```python
from build123d import *

# Parameters (mm, degrees)
SKETCH1_R               = 12.5
SKETCH1_R_2             = 10
BOSS_EXTRUDE1_DEPTH     = 5
SKETCH2_W               = 28
SKETCH2_H               = 28
BOSS_EXTRUDE2_DEPTH     = 25
CUT_EXTRUDE1_DEPTH      = 29
SKETCH7_W               = 9.14199999
SKETCH7_H               = 19.416637146
CUT_EXTRUDE2_DEPTH      = 1
CUT_EXTRUDE2_DEPTH_BACK = 29
SKETCH8_R               = 3.5
CUT_EXTRUDE3_DEPTH      = 1
CUT_EXTRUDE3_DEPTH_BACK = 29


with BuildPart() as part:
    # Sketch1 → Boss-Extrude1 (new body)
    with BuildSketch(Plane.XY):
        Circle(SKETCH1_R)
        Circle(SKETCH1_R_2, mode=Mode.SUBTRACT)
    extrude(amount=BOSS_EXTRUDE1_DEPTH)

    # Sketch2 → Boss-Extrude2 (add)
    with BuildSketch(Plane.XY.offset(5)):
        Rectangle(SKETCH2_W, SKETCH2_H)
    extrude(amount=BOSS_EXTRUDE2_DEPTH)

    # Sketch3 → Cut-Extrude1 (cut, through all)
    with BuildSketch(Plane.ZY.offset(14)):
        with BuildLine():
            Line((17.5, 14), (30, 14))
            Line((30, 14), (30, -14))
            Line((30, -14), (17.5, -14))
            ThreePointArc((17.5, -14), (29.804652609, 0), (17.5, 14))
        make_face()
    extrude(amount=-CUT_EXTRUDE1_DEPTH, mode=Mode.SUBTRACT)

    # Sketch7 → Cut-Extrude2 (cut, two sides)
    with BuildSketch(Plane.XZ.offset(14)) as cut_extrude2_sk:
        with Locations((0, 21.203451283)):
            Rectangle(SKETCH7_W, SKETCH7_H)
    extrude(amount=CUT_EXTRUDE2_DEPTH, mode=Mode.SUBTRACT)
    extrude(cut_extrude2_sk.sketch, amount=-CUT_EXTRUDE2_DEPTH_BACK, mode=Mode.SUBTRACT)

    # Sketch8 → Cut-Extrude3 (cut, two sides)
    with BuildSketch(Plane(origin=(14, 0, 0), x_dir=(0, 0, -1), z_dir=(1, 0, 0))) as cut_extrude3_sk:
        with Locations((-23.652326304, 0)):
            Circle(SKETCH8_R)
    extrude(amount=CUT_EXTRUDE3_DEPTH, mode=Mode.SUBTRACT)
    extrude(cut_extrude3_sk.sketch, amount=-CUT_EXTRUDE3_DEPTH_BACK, mode=Mode.SUBTRACT)


solid = part.part
```
Design review of the part built by this model. Coordinates are the model's own, in mm. A direction names the side the tool comes from. Give positions to 0.01 mm unless a question says otherwise; leave off trailing zeros. Write each loop counter-clockwise with the first axis right and the second up, starting at its lowest first coordinate (ties: lowest second). Pieces come first, ordered by that corner, then holes. Notation, with made-up numbers: (5.5, 52) - (54.5, 52) arc R12 cw to (54.5, 64) - close; hole circle Ø10 at (78.25, 59). An arc over 180 degrees is marked (long way). Return JSON: item names as keys, results as strings. Group by question number.
(1) To check wall thickness, follow probe 1 along X at (y, z) = (7.5, 26.5); probe 2 along Y at (x, z) = (0, 2.4); probe 3 along Z at (x, y) = (4.5, 4.75). State the ranges of each line that lie inside material, in increasing order.
(2) We need section D-D, the plane x = 0. Give the boundary of the cut face in (y, z), then the cut area to 3 significant figures.
(3) We need section C-C, the plane z = 13.25. Give the boundary of the cut face in (x, y).
(4) Insertion check: pin 1 (1 mm diameter, centred on x = -1, y = 5, fed in from -Z); pin 2 (9 mm diameter, centred on y = -1, z = 25, fed in from -X); pin 3 (2.5 mm diameter, centred on x = -1.5, y = 5.5, fed in from +Z); pin 4 (3 mm diameter, centred on x = 4, y = -11, fed in from +Z). Each pin has a flat end and moves straight along its axis. Give the tip position at first contact, or say it passes through.
(5) We need section B-B, the plane z = 21. Give the boundary of the cut face in (x, y).
(6) We need section A-A, the plane y = 0. Give the boundary of the cut face in (x, z).
(7) Machinability: for faces 1 (the flat face through (0, 0, 11.495)), 2 (the flat face through (-13, 0, 5)), 3 (the cylindrical face through (-9.22, 0.15, 27.15)), which of the approach directions +Z, -Z, +X, -X, +Y, -Y give a long, thin tool a straight path to every point of the face, cutting with its end or side? Answer none if there is none.
(8) Mouldability with a two-part tool opening along Y and no side actions: class faces 4 (the flat face through (0, -14, 11)), 5 (the cylindrical face through (9.35, 0.15, 27.15)), 6 (the cylindrical face through (11.923, 3.755, 2.465)) as +Y half, -Y half, draft (parallel to the pull), parting line (faces both ways), or undercut.
Reported:
{
 "1": {"probe 1": "x = -14 to -4.57, 4.57 to 14", "probe 2": "y = -12.5 to -10, 10 to 12.5", "probe 3": "z = 5 to 11.5"},
 "2": {"outline": "(-14, 5) - (-12.5, 5) - (-12.5, 0) - (-10, 0) - (-10, 5) - (10, 5) - (10, 0) - (12.5, 0) - (12.5, 5) - (14, 5) - (14, 11.5) - (-14, 11.5) - close", "area": "207 mm2"},
 "3": {"outline": "(-14, -14) - (-4.57, -14) - (-4.57, 14) - (-14, 14) - close; (4.57, -14) - (14, -14) - (14, 14) - (4.57, 14) - close"},
 "4": {"pin 1": "stops at z = 5", "pin 2": "stops at x = -14", "pin 3": "stops at z = 11.5", "pin 4": "stops at z = 26.03"},
 "5": {"outline": "(-14, -13.08) - (-4.57, -13.08) - (-4.57, -2.28) - (-14, -2.28) - close; (-14, 2.28) - (-4.57, 2.28) - (-4.57, 13.08) - (-14, 13.08) - close; (4.57, -13.08) - (14, -13.08) - (14, -2.28) - (4.57, -2.28) - close; (4.57, 2.28) - (14, 2.28) - (14, 13.08) - (4.57, 13.08) - close"},
 "6": {"outline": "(-14, 5) - (-12.5, 5) - (-12.5, 0) - (-10, 0) - (-10, 5) - (10, 5) - (10, 0) - (12.5, 0) - (12.5, 5) - (14, 5) - (14, 20.15) - (4.57, 20.15) - (4.57, 11.5) - (-4.57, 11.5) - (-4.57, 20.15) - (-14, 20.15) - close; (-14, 27.15) - (-4.57, 27.15) - (-4.57, 29.8) - (-14, 29.8) - close; (4.57, 27.15) - (14, 27.15) - (14, 29.8) - (4.57, 29.8) - close"},
 "7": {"face 1": "+Z, +Y, -Y", "face 2": "-Z", "face 3": "+X, -X"},
 "8": {"face 4": "-Y half", "face 5": "undercut", "face 6": "parting line"}
}
